from build123d import *

# Parameters (mm, degrees)
SKETCH1_W           = 24
SKETCH1_H           = 48
BOSS_EXTRUDE1_DEPTH = 2
SKETCH2_R           = 1
CUT_EXTRUDE1_DEPTH  = 2
SKETCH3_R           = 1.6
CUT_EXTRUDE2_DEPTH  = 2
SKETCH5_W           = 4.002629444
SKETCH5_H           = 28.892829006
BOSS_EXTRUDE2_DEPTH = 3
SKETCH7_W           = 4.002629444
SKETCH7_H           = 6.221455563
CUT_EXTRUDE3_DEPTH  = 3
SKETCH8_W           = 10.000621013
SKETCH8_H           = 3.995270277
SKETCH8_W_2         = 9.996749543
BOSS_EXTRUDE3_DEPTH = 3
SKETCH9_W           = 24
SKETCH9_H           = 2
CUT_EXTRUDE4_DEPTH  = 4


with BuildPart() as part:
    # Sketch1 → Boss-Extrude1 (new body)
    with BuildSketch(Plane(origin=(0, 0, 0), x_dir=(1, 0, 0), z_dir=(0, 1, 0))):
        with Locations((12, 24)):
            Rectangle(SKETCH1_W, SKETCH1_H)
    extrude(amount=BOSS_EXTRUDE1_DEPTH)

    # Sketch2 → Cut-Extrude1 (cut)
    with BuildSketch(Plane(origin=(0, 2, 0), x_dir=(1, 0, 0), z_dir=(0, 1, 0))):
        with Locations(Location((2.995742756, 45.004810193, 0), (0, 0, 270))):
            Circle(SKETCH2_R)
        with Locations(Location((21.000528316, 45.004810193, 0), (0, 0, 270))):
            Circle(SKETCH2_R)
    extrude(amount=-CUT_EXTRUDE1_DEPTH, mode=Mode.SUBTRACT)

    # Sketch3 → Cut-Extrude2 (cut)
    with BuildSketch(Plane(origin=(0, 2, 0), x_dir=(1, 0, 0), z_dir=(0, 1, 0))):
        with Locations((2.997154371, 14.995076851)):
            Circle(SKETCH3_R)
        with Locations((2.997154371, 16.595076851)):
            Circle(SKETCH3_R)
        with Locations((2.997154371, 13.395076851)):
            Circle(SKETCH3_R)
        with BuildLine():
            ThreePointArc((1.611513725, 15.795076851), (1.451673049, 16.180966379), (1.397154371, 16.595076851))
            Line((1.397154371, 16.595076851), (1.397154371, 14.995076851))
            ThreePointArc((1.397154371, 14.995076851), (1.451673049, 15.409187323), (1.611513725, 15.795076851))
        make_face()
        with BuildLine():
            ThreePointArc((1.611513725, 14.195076851), (1.451673049, 14.580966379), (1.397154371, 14.995076851))
            Line((1.397154371, 14.995076851), (1.397154371, 13.395076851))
            ThreePointArc((1.397154371, 13.395076851), (1.451673049, 13.809187323), (1.611513725, 14.195076851))
        make_face()
        with BuildLine():
            Line((4.597154371, 13.395076851), (4.597154371, 14.995076851))
            ThreePointArc((4.597154371, 14.995076851), (4.542635694, 14.580966379), (4.382795018, 14.195076851))
            ThreePointArc((4.382795018, 14.195076851), (4.542635694, 13.809187323), (4.597154371, 13.395076851))
        make_face()
        with BuildLine():
            Line((4.597154371, 14.995076851), (4.597154371, 16.595076851))
            ThreePointArc((4.597154371, 16.595076851), (4.542635694, 16.180966379), (4.382795018, 15.795076851))
            ThreePointArc((4.382795018, 15.795076851), (4.542635694, 15.409187323), (4.597154371, 14.995076851))
        make_face()
        with Locations((21.000046924, 14.995076851)):
            Circle(SKETCH3_R)
        with Locations((21.000046924, 16.595076851)):
            Circle(SKETCH3_R)
        with Locations((21.000046924, 13.395076851)):
            Circle(SKETCH3_R)
        with BuildLine():
            Line((22.600046924, 13.395076851), (22.600046924, 14.995076851))
            ThreePointArc((22.600046924, 14.995076851), (22.545528247, 14.580966379), (22.385687571, 14.195076851))
            ThreePointArc((22.385687571, 14.195076851), (22.545528247, 13.809187323), (22.600046924, 13.395076851))
        make_face()
        with BuildLine():
            Line((22.600046924, 14.995076851), (22.600046924, 16.595076851))
            ThreePointArc((22.600046924, 16.595076851), (22.545528247, 16.180966379), (22.385687571, 15.795076851))
            ThreePointArc((22.385687571, 15.795076851), (22.545528247, 15.409187323), (22.600046924, 14.995076851))
        make_face()
        with BuildLine():
            ThreePointArc((19.614406278, 15.795076851), (19.454565602, 16.180966379), (19.400046924, 16.595076851))
            Line((19.400046924, 16.595076851), (19.400046924, 14.995076851))
            ThreePointArc((19.400046924, 14.995076851), (19.454565602, 15.409187323), (19.614406278, 15.795076851))
        make_face()
        with BuildLine():
            ThreePointArc((19.614406278, 14.195076851), (19.454565602, 14.580966379), (19.400046924, 14.995076851))
            Line((19.400046924, 14.995076851), (19.400046924, 13.395076851))
            ThreePointArc((19.400046924, 13.395076851), (19.454565602, 13.809187323), (19.614406278, 14.195076851))
        make_face()
    extrude(amount=-CUT_EXTRUDE2_DEPTH, mode=Mode.SUBTRACT)

    # Sketch5 → Boss-Extrude2 (add)
    with BuildSketch(Plane(origin=(0, 0, 0), x_dir=(-1, 0, 0), z_dir=(0, -1, 0))):
        with Locations((-11.998064265, 33.553585497)):
            Rectangle(SKETCH5_W, SKETCH5_H)
    extrude(amount=BOSS_EXTRUDE2_DEPTH)

    # Sketch7 → Cut-Extrude3 (cut)
    with BuildSketch(Plane(origin=(0, -3, 0), x_dir=(-1, 0, 0), z_dir=(0, -1, 0))):
        with Locations((-11.998064265, 44.889272218)):
            Rectangle(SKETCH7_W, SKETCH7_H)
    extrude(amount=-CUT_EXTRUDE3_DEPTH, mode=Mode.SUBTRACT)

    # Sketch8 → Boss-Extrude3 (add)
    with BuildSketch(Plane(origin=(0, 0, 0), x_dir=(-1, 0, 0), z_dir=(0, -1, 0))):
        with Locations((-18.999689494, 39.780909299)):
            Rectangle(SKETCH8_W, SKETCH8_H)
        with Locations((-4.998374771, 39.780909299)):
            Rectangle(SKETCH8_W_2, SKETCH8_H)
    extrude(amount=BOSS_EXTRUDE3_DEPTH)

    # Sketch9 → Cut-Extrude4 (cut)
    with BuildSketch(Plane.XY):
        with Locations((12, 1)):
            Rectangle(SKETCH9_W, SKETCH9_H)
    extrude(amount=-CUT_EXTRUDE4_DEPTH, mode=Mode.SUBTRACT)


solid = part.part
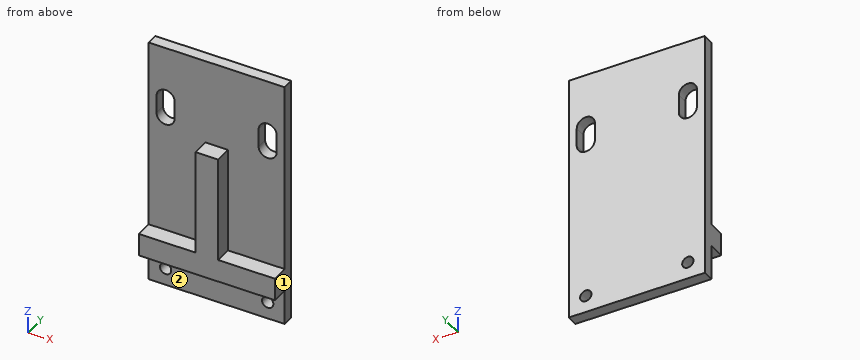
CAD build for the part. Positions are in the model's coordinates, mm. Face numbers are marked on the shaded views. A direction names the side the tool comes from. Round coordinates to 2 decimals unless told otherwise and drop trailing zeros. Write each loop counter-clockwise with the first axis right and the second up, starting at its lowest first coordinate (ties: lowest second). Pieces come first, ordered by that corner, then holes. Notation, with made-up numbers: M 48.25,3 L 54.25,3 A28 ccw 54.25,22 Z; hole C 89,83 d10. An arc over 180 degrees is marked long. Use a Markdown table: item, result. Add a question column.
1. Flat gauge pins, fed straight in: P1, Ø1, axis at x = 3, z = -29, coming from the -Y side; P2, Ø2.5, axis at x = 6.5, y = -1.5, coming from the -Z side; P3, Ø0.9, axis at x = 5, y = -1.5, coming from the +Z side. Where does each tip first touch, or does it go through?
2. Drill centre lines: probe 1 along X at (y, z) = (0.9, -16); probe 2 along Z at (x, y) = (3.75, 0.4); probe 3 along Z at (x, y) = (20.5, 1.75). Where is each one in solid material? Low to high.
3. Slice it at A-A on z = -17.5. Give the cut face in (x, y), then the cut area to 3 significant figures.
4. Slice it at C-C on y = -2.3. Give the cut face in (x, z).
5. Slice it at B-B on x = 3.5. Give the cut face in (y, z), then the cut area to 3 significant figures.
6. Slice it at D-D on x = 8. Give the cut face in (y, z), then the cut area to 4 significant figures.
7. 3-axis set-ups, long thin cutter, end or side, ignore diameter. For the marked faces 1 and 2: which of +Z, -Z, +X, -X, +Y, -Y reach the whole face in a straight line?
Reply:
| question | item | result |
|---|---|---|
| 1 | P1 | stops at y = 0 |
| 1 | P2 | stops at z = -41.78 |
| 1 | P3 | stops at z = -37.78 |
| 2 | probe 1 | x = 0 to 1.4, 4.6 to 19.4, 22.6 to 24 |
| 2 | probe 2 | z = -48 to -45.66, -44.35 to -18.01, -11.98 to -4 |
| 2 | probe 3 | z = -48 to -45.87, -44.14 to -18.11, -11.88 to -4 |
| 3 | outline | M 0,0 L 1.68,0 L 1.68,2 L 0,2 Z; M 4.32,0 L 19.68,0 L 19.68,2 L 4.32,2 Z; M 22.32,0 L 24,0 L 24,2 L 22.32,2 Z |
| 3 | area | 37.4 mm^2 |
| 4 | outline | M 0,-41.78 L 24,-41.78 L 24,-37.78 L 14,-37.78 L 14,-19.11 L 10,-19.11 L 10,-37.78 L 0,-37.78 Z |
| 5 | outline | M -3,-41.78 L 0,-41.78 L 0,-44.14 L 2,-44.14 L 2,-18.11 L 0,-18.11 L 0,-37.78 L -3,-37.78 Z; M 0,-48 L 2,-48 L 2,-45.87 L 0,-45.87 Z; M 0,-11.88 L 2,-11.88 L 2,-4 L 0,-4 Z |
| 5 | area | 84.1 mm^2 |
| 6 | outline | M -3,-41.78 L 0,-41.78 L 0,-48 L 2,-48 L 2,-4 L 0,-4 L 0,-37.78 L -3,-37.78 Z |
| 6 | area | 100.0 mm^2 |
| 7 | face 1 | +Z, -Z, +X, +Y, -Y |
| 7 | face 2 | -Z, +X, -X, -Y |
